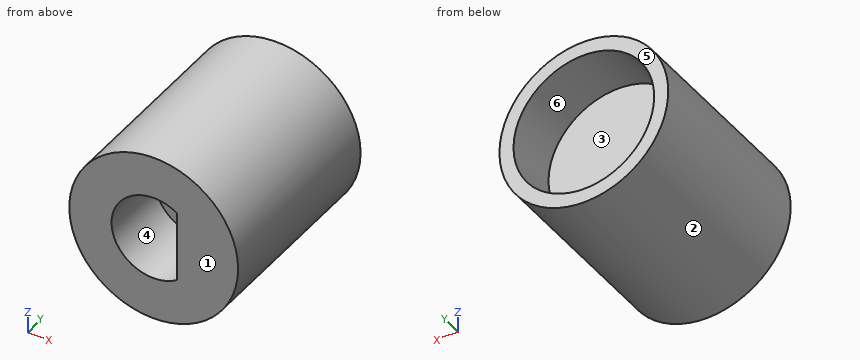
from build123d import *

# Parameters (mm, degrees)
SKETCH_1_R          = 3
EXTRUDE_1_DEPTH     = 7
CUT_EXTRUDE_1_DEPTH = 2.5
SKETCH_5_R          = 2.5
CUT_EXTRUDE_2_DEPTH = 2


with BuildPart() as part:
    # 草图1 → 凸台-拉伸1 (new body)
    with BuildSketch(Plane(origin=(0, 0, 0), x_dir=(1, 0, 0), z_dir=(0, 1, 0))):
        Circle(SKETCH_1_R)
    extrude(amount=EXTRUDE_1_DEPTH)

    # 草图4 → 切除-拉伸1 (cut)
    with BuildSketch(Plane(origin=(0, 0, 0), x_dir=(1, 0, 0), z_dir=(0, 1, 0))):
        with BuildLine():
            Line((0.829156198, -1.25), (0.829156198, 1.25))
            ThreePointArc((0.829156198, 1.25), (-1.5, 0), (0.829156198, -1.25))
        make_face()
    extrude(amount=CUT_EXTRUDE_1_DEPTH, mode=Mode.SUBTRACT)

    # 草图5 → 切除-拉伸2 (cut)
    with BuildSketch(Plane(origin=(0, 7, 0), x_dir=(1, 0, 0), z_dir=(0, 1, 0))):
        Circle(SKETCH_5_R)
    extrude(amount=-CUT_EXTRUDE_2_DEPTH, mode=Mode.SUBTRACT)


solid = part.part
Model file for the job. Use its own axes, mm. Face numbers are marked on the shaded views. A direction names the side the tool comes from. Round coordinates to 2 decimals unless told otherwise and drop trailing zeros. Loops run counter-clockwise (first coordinate to the right, second up) from the corner with the lowest first, then second, coordinate; pieces in that order, holes last. Notation, with made-up numbers: M 67.5,26 L 108.5,26 A27 ccw 108.5,49 Z; hole C 14,63.5 d1. An arc over 180 degrees is marked long. One line per question, with ' | ' between items.
1) Band-saw the part on A-A (x = 0). Give the cut face in (y, z), then the cut area to 3 significant figures.
Solved:
outline: M 0,-3 L 7,-3 L 7,-2.5 L 5,-2.5 L 5,2.5 L 7,2.5 L 7,3 L 0,3 L 0,1.5 L 2.5,1.5 L 2.5,-1.5 L 0,-1.5 Z | area: 24.5 mm²
2) Band-saw the part on B-B (z = 0). Give the cut face in (x, y), then the cut area to 3 significant figures.
Solved:
outline: M -3,0 L -1.5,0 L -1.5,2.5 L 0.83,2.5 L 0.83,0 L 3,0 L 3,7 L 2.5,7 L 2.5,5 L -2.5,5 L -2.5,7 L -3,7 Z | area: 26.2 mm²
3) Mould opens along Z. For the marked faces 1, 2 and 3 say: +Z half, -Z half, draft (parallel to the pull), parting line (faces both ways), or undercut.
Solved:
face 1: draft | face 2: parting line | face 3: undercut
4) Flat gauge pins, fed straight in: pin 1 (1.5 mm diameter, centred on x = -0.5, z = -1, fed in from +Y); pin 2 (1.5 mm diameter, centred on y = 3, z = 1.5, fed in from -X); pin 3 (0.7 mm diameter, centred on x = -0.5, z = 0.5, fed in from -Y). Where does each tip first touch, or does it go through?
Solved:
pin 1: stops at y = 5 | pin 2: stops at x = -2.9 | pin 3: stops at y = 2.5
5) Band-saw the part on D-D (y = 3.75). Give the cut face in (x, z).
Solved:
outline: C 0,0 d6
6) Drill centre lines: line 1 along Z through (x, y) = (0, 5.85); line 2 along Z through (x, y) = (0, 1.05). Where is each one in solid material? Low to high.
Solved:
line 1: z = -3 to -2.5, 2.5 to 3 | line 2: z = -3 to -1.5, 1.5 to 3
7) Band-saw the part on C-C (y = 0.5). Give the cut face in (x, z), then the cut area to 3 significant figures.
Solved:
outline: C 0,0 d6; hole M 0.83,-1.25 L 0.83,1.25 A1.5 ccw long Z | area: 22.4 mm²
8) 3-axis set-ups, long thin cutter, end or side, ignore diameter. For the marked faces 4, 5 and 6: which of +Z, -Z, +X, -X, +Y, -Y reach the whole face in a straight line?
Solved:
face 4: -Y | face 5: +Z, -Z, +X, -X, +Y | face 6: +Y
